Can you work these out from the drawing? Everything is in mm from the part's minimum corner. Coordinates: 2 decimals unless noted, no trailing zeros. Loops run counter-clockwise (first coordinate to the right, second up) from the corner with the lowest first, then second, coordinate; pieces in that order, holes last.
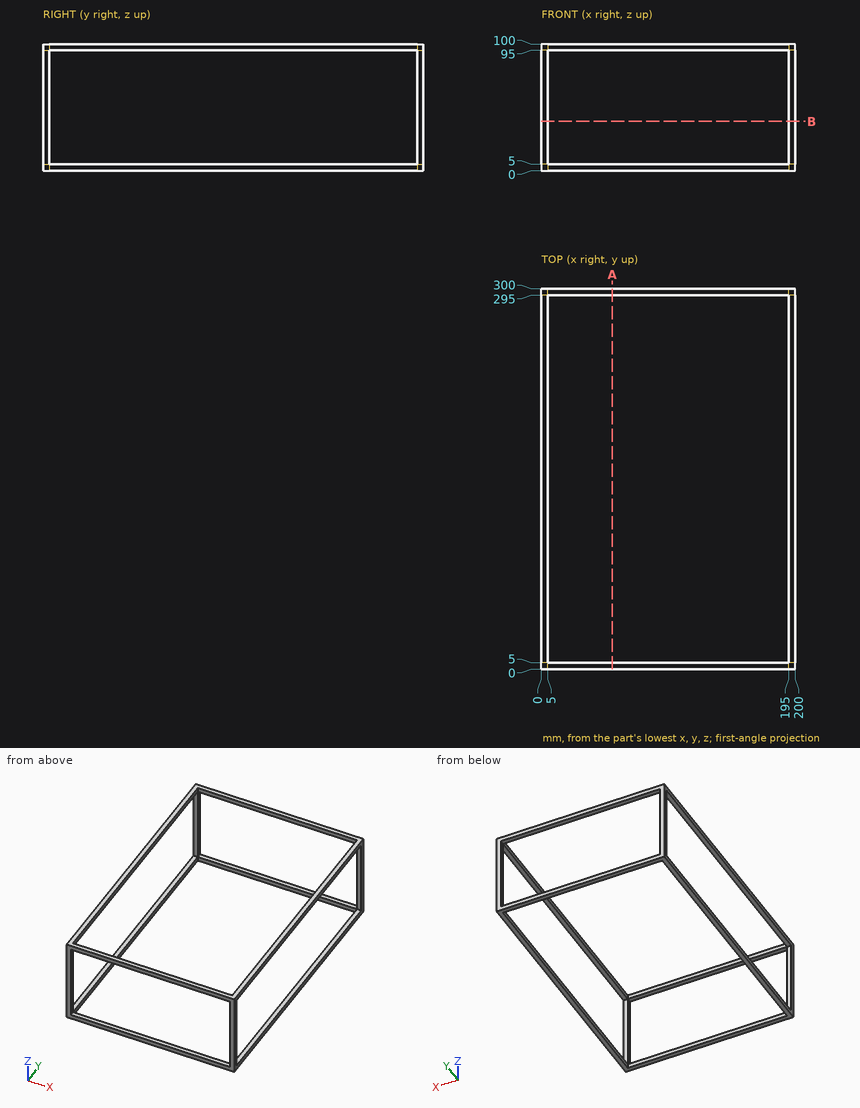
Item 1: I need wall thicknesses on line 1 along Y through (x, z) = (122, 95.5). Which ranges of the line are inside material? Lowest first, please.
Results are:
line 1: y = 0 to 5, 295 to 300
Item 2: Suppose I cut it at B-B, the plane z = 39. Please give me the cut outline in (x, y), plus the area to 3 significant figures.
Results are:
outline: (0, 0) - (5, 0) - (5, 5) - (0, 5) - close; (0, 295) - (5, 295) - (5, 300) - (0, 300) - close; (195, 0) - (200, 0) - (200, 5) - (195, 5) - close; (195, 295) - (200, 295) - (200, 300) - (195, 300) - close
area: 100 mm2
Item 3: Suppose I cut it at A-A, the plane x = 56. Please give me the cut outline in (y, z).
Results are:
outline: (0, 0) - (5, 0) - (5, 5) - (0, 5) - close; (0, 95) - (5, 95) - (5, 100) - (0, 100) - close; (295, 0) - (300, 0) - (300, 5) - (295, 5) - close; (295, 95) - (300, 95) - (300, 100) - (295, 100) - close
Item 4: I'm going to push a flat-ended pin straight in: P1, Ø4, axis at x = 198, y = 83, coming from the -Z side. Where does the tip first touch, or does it pass through?
Results are:
P1: stops at z = 0
